Geometry check sheet. Reference: the model listing, model coordinates, mm. A direction names the side the tool comes from. Coordinates: 2 decimals unless noted, no trailing zeros. Write each loop counter-clockwise with the first axis right and the second up, starting at its lowest first coordinate (ties: lowest second). Pieces come first, ordered by that corner, then holes. Notation, with made-up numbers: (50.5, 52) -> (83.5, 52) arc R30 cw to (83.5, 86) -> close; hole circle Ø11 at (43.5, -0.5). An arc over 180 degrees is marked (long way). Answer in a Markdown table with one row per item. Add a question column.
1. Set-up check for faces 1 (the flat face through (13, -8.382, 1)), 2 (the flat face through (-10.6, -8.382, 0.8)), 3 (the flat face through (11.048, -30, 1)), 4 (the cylindrical face through (-1.24, -8.11, 0.83)): record each of +Z, -Z, +X, -X, +Y, -Y from which the full face is reachable in a straight line by a thin tool's end or side.
2. Cross-section at A-A on y = -3.5. Record the cut outline in (x, z).
3. Cross-section at B-B on y = -9. Record the cut outline in (x, z), and give its area (3 significant figures).
4. Mould release check, pull along X, two halves, no side actions. Record for faces 5 (the flat face through (10.16, -4, 1)), 6 (the flat face through (0, -15, 0)), 7 (the flat face through (11.048, -9, 1)): pulls with the +X half, pulls with the -X half, needs draft (parallel to the pull), parting line crosses it, or undercut.
5. Scan lines: L1, parallel to X at y = -1.5, z = 1; L2, parallel to Y at x = 13, z = 0.75; L3, parallel to Y at x = -11.5, z = 1.55. Record each from-to range of solid material in increasing order. Write a range as from..to.
6. Depth check by flat-ended pin: P1, Ø0.8, axis at x = -13, z = 0.5, coming from the +Y side; P2, Ø0.5, axis at y = -6.5, z = 1, coming from the -X side. Enter the tip coordinate at first touch or a pass-through.
```python
from build123d import *

# Parameters (mm, degrees)
F0_W     = 28.321
F0_H     = 30.48
F1_DEPTH = 1.64
F2_W     = 1.905
F2_H     = 8.382
F2_W_2   = 1.207
F2_H_2   = 1.5875
F3_DEPTH = 25
F4_R     = 0.95249
F5_SIZE  = 0.507
F6_R     = 0.60349


# Not quite as in the source:
# - a fillet or chamfer is up to 0.001 mm smaller than in the source, because OpenCascade refuses the exact size


with BuildPart() as f1:
    # F0 (on Top) → F1 (new body)
    with BuildSketch(Plane.XY):
        with Locations((0, -15.24)):
            Rectangle(F0_W, F0_H)
    extrude(amount=F1_DEPTH)

    # F2 (on Top) → F3 (cut)
    with BuildSketch(Plane.XY):
        Polygon((-10.1605, 0), (-14.1605, 0), (-14.1605, -8.382), (-12.2555, -8.382), (-12.2555, -9.9695), (-11.0485, -9.9695), (-11.0485, -8.382), (-10.1605, -8.382), align=None)
        with Locations((-1.905, -4.191)):
            Rectangle(F2_W, F2_H)
        Polygon((14.1605, -8.382), (14.1605, 0), (10.1595, 0), (10.1595, -8.382), (11.0485, -8.382), (11.0485, -9.9695), (12.2555, -9.9695), (12.2555, -8.382), align=None)
        with Locations((-11.652, -29.68625)):
            Rectangle(F2_W_2, F2_H_2)
        with Locations((11.652, -29.68625)):
            Rectangle(F2_W_2, F2_H_2)
    extrude(amount=F3_DEPTH, mode=Mode.SUBTRACT)

    # F4 (radius 0.9525 in the source; OpenCascade refuses exactly that, so slightly less here)
    f4_edges = [f1.edges().sort_by_distance(p)[0] for p in [
        (-2.8575, -8.382, 0.82),
        (-0.9525, -8.382, 0.82),
    ]]
    fillet(f4_edges, radius=F4_R)

    # F5
    f5_edges = [f1.edges().sort_by_distance(p)[0] for p in [
        (10.1595, 0, 0.82),
        (-0.9525, 0, 0.82),
        (-2.8575, 0, 0.82),
        (-10.1605, 0, 0.82),
    ]]
    chamfer(f5_edges, length=F5_SIZE)

    # F6 (radius 0.6035 in the source; OpenCascade refuses exactly that, so slightly less here)
    f6_edges = [f1.edges().sort_by_distance(p)[0] for p in [
        (12.2555, -28.8925, 0.82),
        (-12.2555, -28.8925, 0.82),
        (-11.0485, -28.8925, 0.82),
        (11.0485, -28.8925, 0.82),
        (11.0485, -9.9695, 0.82),
        (12.2555, -9.9695, 0.82),
        (-12.2555, -9.9695, 0.82),
        (-11.0485, -9.9695, 0.82),
    ]]
    fillet(f6_edges, radius=F6_R)


solid = f1.part
```
Results found:
| question | item | result |
|---|---|---|
| 1 | face 1 | +Z, -Z, +X, +Y |
| 1 | face 2 | +Z, -Z, -X, +Y |
| 1 | face 3 | +Z, -Z, -Y |
| 1 | face 4 | +Z, -Z, +Y |
| 2 | outline | (-10.16, 0) -> (-2.86, 0) -> (-2.86, 1.64) -> (-10.16, 1.64) -> close; (-0.95, 0) -> (10.16, 0) -> (10.16, 1.64) -> (-0.95, 1.64) -> close |
| 3 | outline | (-14.16, 0) -> (-12.26, 0) -> (-12.26, 1.64) -> (-14.16, 1.64) -> close; (-11.05, 0) -> (11.05, 0) -> (11.05, 1.64) -> (-11.05, 1.64) -> close; (12.26, 0) -> (14.16, 0) -> (14.16, 1.64) -> (12.26, 1.64) -> close |
| 3 | area | 42.5 mm^2 |
| 4 | face 5 | pulls with the +X half |
| 4 | face 6 | needs draft |
| 4 | face 7 | undercut |
| 5 | L1 | x = -10.16..-2.86, -0.95..10.16 |
| 5 | L2 | y = -30.48..-8.38 |
| 5 | L3 | y = -28.91..-9.95 |
| 6 | P1 | stops at y = -8.38 |
| 6 | P2 | stops at x = -10.16 |
